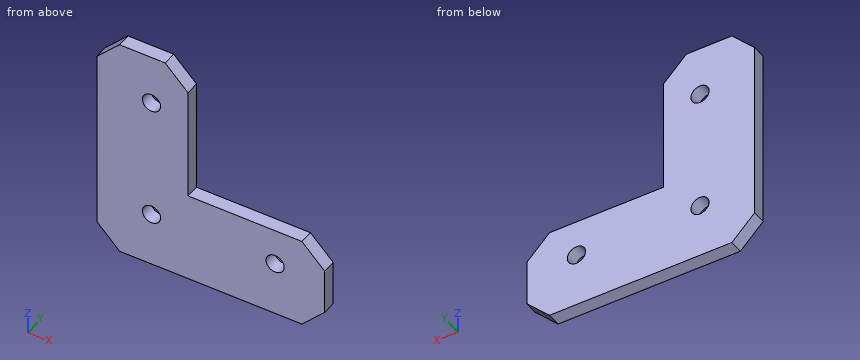
```python
from build123d import *

# Parameters (mm, degrees)
F0_R     = 2
F1_DEPTH = 3
F2_SIZE  = 5


with BuildPart() as f1:
    # F0 (on Front) → F1 (new body)
    with BuildSketch(Plane.XZ):
        Polygon((-35.773953, 50), (-55.773953, 50), (-55.773953, 0), (-5.773953, 0), (-5.773953, 20), (-35.773953, 20), align=None)
        with Locations((-43.773953, 12)):
            Circle(F0_R, mode=Mode.SUBTRACT)
        with Locations((-16.65267, 12)):
            Circle(F0_R, mode=Mode.SUBTRACT)
        with Locations((-43.773953, 38.991082)):
            Circle(F0_R, mode=Mode.SUBTRACT)
    extrude(amount=F1_DEPTH)

    # F2
    f2_edges = [f1.edges().sort_by_distance(p)[0] for p in [
        (-55.773953, -1.5, 50),
        (-35.773953, -1.5, 50),
        (-5.773953, -1.5, 20),
        (-5.773953, -1.5, 0),
        (-55.773953, -1.5, 0),
    ]]
    chamfer(f2_edges, length=F2_SIZE)


solid = f1.part
```
The listing builds one solid part. Answer for the finished solid, in the listing's coordinates (mm). Round coordinates to 2 decimals unless told otherwise and drop trailing zeros. Order: outer loops, then holes, each group sorted by start corner. A loop starts at its lowest first (then second) coordinate and runs counter-clockwise, first axis right, second up. Notation, with made-up numbers: (-5, -40) - (11, -40) arc R24 cw to (11, -11) - close; hole circle Ø2 at (-19, 13). An arc over 180 degrees is marked (long way). Put each result on its own line as item: value. Start each with the question number.
(1) Find section B-B (x = -18). Give the vertices of the cut face in (y, z), plus the area to 3 significant figures.
(2) Find section D-D (z = 32.5). Give the vertices of the cut face in (x, y).
(3) Find section A-A (z = 12). Give the vertices of the cut face in (x, y).
(4) Find section C-C (y = -2.25). Give the vertices of the cut face in (x, z), plus the area to 3 significant figures.
(5) Straight lines are drawn through the part: probe 1 along X at (y, z) = (-1.1, 13); probe 2 along Z at (x, y) = (-28, -2.05); probe 3 along X at (y, z) = (-1.45, 43.5). For each, find the intervals that lie inside material, in ascending order. Write a range as from..to.
(6) Given P1, Ø2.5, axis at x = -43.77, z = 12, coming from the -Y side; P2, Ø0.9, axis at y = -2, z = 35.5, coming from the +X side; P3, Ø6.5, axis at x = -43.77, z = 38.99, coming from the +Y side, each flat-ended and moving along its own axis, determine where each tip first touches the part or whether it passes through.
Reply:
1. outline: (-3, 0) - (0, 0) - (0, 10.52) - (-3, 10.52) - close; (-3, 13.48) - (0, 13.48) - (0, 20) - (-3, 20) - close
1. area: 51.1 mm^2
2. outline: (-55.77, -3) - (-35.77, -3) - (-35.77, 0) - (-55.77, 0) - close
3. outline: (-55.77, -3) - (-45.77, -3) - (-45.77, 0) - (-55.77, 0) - close; (-41.77, -3) - (-18.65, -3) - (-18.65, 0) - (-41.77, 0) - close; (-14.65, -3) - (-5.77, -3) - (-5.77, 0) - (-14.65, 0) - close
4. outline: (-55.77, 5) - (-50.77, 0) - (-10.77, 0) - (-5.77, 5) - (-5.77, 15) - (-10.77, 20) - (-35.77, 20) - (-35.77, 45) - (-40.77, 50) - (-50.77, 50) - (-55.77, 45) - close; hole circle Ø4 at (-43.77, 12); hole circle Ø4 at (-43.77, 38.99); hole circle Ø4 at (-16.65, 12)
4. area: 1,500 mm^2
5. probe 1: -55.77..-45.51, -42.04..-18.38, -14.92..-5.77
5. probe 2: 0..20
5. probe 3: -55.77..-35.77
6. P1: through
6. P2: x = -35.77
6. P3: y = 0
